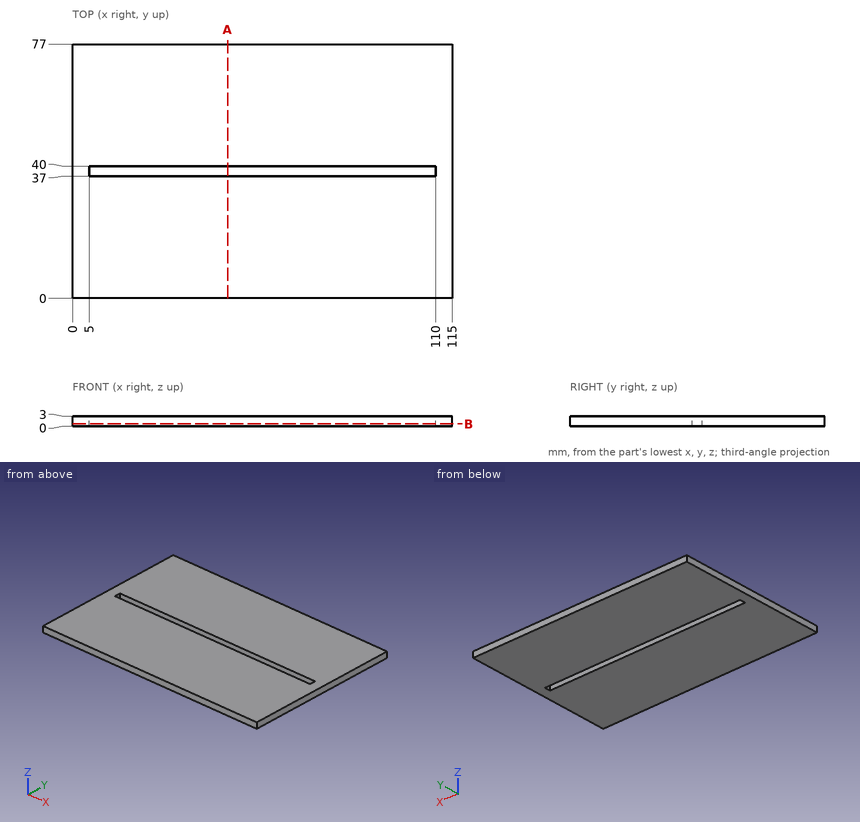
Verification items for this drawing (mm, ordinates from the low corner). Give positions to 0.01 mm unless a question says otherwise; leave off trailing zeros. Loops run counter-clockwise (first coordinate to the right, second up) from the corner with the lowest first, then second, coordinate; pieces in that order, holes last. Notation, with made-up numbers: M 2.5,-2 L 24.5,-2 A19 cw 24.5,27 Z; hole C -5,-29.5 d5. An arc over 180 degrees is marked long. Return JSON: item names as keys, results as strings. Group by question number.
1. Cross-section at B-B on z = 0.7. Record the boundary of the cut face in (x, y), plus the area to 3 significant figures.
2. Cross-section at A-A on x = 47. Record the boundary of the cut face in (y, z), plus the area to 3 significant figures.
3. Thickness scan on L1, parallel to Y at x = 51, z = 1.5; L2, parallel to X at y = 38.5, z = 0.55. Record the ranges inside material, lowest first.
Return value:
{
 "1": {"outline": "M 0,0 L 115,0 L 115,77 L 0,77 Z; hole M 5,37 L 110,37 L 110,40 L 5,40 Z", "area": "8,540 mm^2"},
 "2": {"outline": "M 0,0 L 37,0 L 37,3 L 0,3 Z; M 40,0 L 77,0 L 77,3 L 40,3 Z", "area": "222 mm^2"},
 "3": {"L1": "0 to 37, 40 to 77", "L2": "0 to 5, 110 to 115"}
}
